```python
from build123d import *
from build123d.topology import SkipClean

# Parameters (mm, degrees)
EXTRUDE1_DEPTH  = 21.397127
SKETCH4_W       = 60
SKETCH4_H       = 29.397126503
SKETCH3_W       = 80
SKETCH3_H       = 20
EXTRUDE2_DEPTH  = 10
EXTRUDE3_DEPTH  = 9
SKETCH7_W       = 60.014196904
SKETCH7_H       = 26.778889024
EXTRUDE4_DEPTH  = 11
SKETCH8_W       = 71.467077652
SKETCH8_H       = 25.017155062
EXTRUDE5_DEPTH  = 23
SKETCH9_W       = 59.977554146
SKETCH9_H       = 30.874003366
EXTRUDE6_DEPTH  = 7
SKETCH10_R      = 2.5
EXTRUDE7_DEPTH  = 65
SKETCH12_R      = 5
EXTRUDE8_DEPTH  = 65
SKETCH13_R      = 2.15
EXTRUDE9_DEPTH  = 65
SKETCH14_R      = 4
EXTRUDE10_DEPTH = 65


with BuildPart() as part:
    # Sketch1 → Extrude1 (new body)
    with BuildSketch(Plane.XY):
        with BuildLine():
            Line((-96.138674094, 82.333988555), (-46.138674094, 82.333988555))
            Line((-46.138674094, 82.333988555), (-46.138674094, 131.333988555))
            ThreePointArc((-46.138674094, 131.333988555), (-47.017353751, 133.455308898), (-49.138674094, 134.333988555))
            Line((-49.138674094, 134.333988555), (-93.138674094, 134.333988555))
            ThreePointArc((-93.138674094, 134.333988555), (-95.259994438, 133.455308898), (-96.138674094, 131.333988555))
            Line((-96.138674094, 131.333988555), (-96.138674094, 82.333988555))
        make_face()
        with BuildLine():
            ThreePointArc((-86.138674094, 92.833988555), (-83.638674094, 95.333988555), (-86.138674094, 97.833988555))
            ThreePointArc((-86.138674094, 97.833988555), (-88.638674094, 95.333988555), (-86.138674094, 92.833988555))
        make_face(mode=Mode.SUBTRACT)
        with BuildLine():
            ThreePointArc((-56.138674094, 92.833988555), (-53.638674094, 95.333988555), (-56.138674094, 97.833988555))
            ThreePointArc((-56.138674094, 97.833988555), (-58.638674094, 95.333988555), (-56.138674094, 92.833988555))
        make_face(mode=Mode.SUBTRACT)
        with BuildLine():
            ThreePointArc((-86.138674094, 127.833988555), (-88.638674094, 125.333988555), (-86.138674094, 122.833988555))
            ThreePointArc((-86.138674094, 122.833988555), (-83.638674094, 125.333988555), (-86.138674094, 127.833988555))
        make_face(mode=Mode.SUBTRACT)
        with BuildLine():
            ThreePointArc((-56.138674094, 122.833988555), (-53.638674094, 125.333988555), (-56.138674094, 127.833988555))
            ThreePointArc((-56.138674094, 127.833988555), (-58.638674094, 125.333988555), (-56.138674094, 122.833988555))
        make_face(mode=Mode.SUBTRACT)
        with BuildLine():
            ThreePointArc((-71.138674094, 125.333988555), (-86.138674094, 110.333988555), (-71.138674094, 95.333988555))
            ThreePointArc((-71.138674094, 95.333988555), (-56.138674094, 110.333988555), (-71.138674094, 125.333988555))
        make_face(mode=Mode.SUBTRACT)
    extrude(amount=EXTRUDE1_DEPTH)

    # Sketch4 → Loft1 section 0
    with BuildSketch(Plane(origin=(0, 117.333988555, 0), x_dir=(1, 0, 0), z_dir=(0, 1, 0))):
        with Locations((-71.138674094, -14.698563252)):
            Rectangle(SKETCH4_W, SKETCH4_H)
    # Sketch3 → Loft1 section 1
    with BuildSketch(Plane(origin=(0, 102.333988555, 0), x_dir=(1, 0, 0), z_dir=(0, 1, 0))):
        with Locations((-71.138674094, -31.397126503)):
            Rectangle(SKETCH3_W, SKETCH3_H)
    loft()

    # Sketch5 → Extrude2 (add)
    with BuildSketch(Plane(origin=(25.673528037, 17.115685358, 0), x_dir=(0, 0, -1), z_dir=(0.8320502943378439, 0.5547001962252289, 0))):
        Polygon((-29.397126503, 120.447410305), (-15.115551494, 141.902806552), (0, 141.902806552), (0, 120.447410305), align=None)
    extrude2 = extrude(amount=-EXTRUDE2_DEPTH)

    # Mirror1: Extrude2 across plane
    add(extrude2.mirror(Plane(origin=(-71.138674094, 0, 0), x_dir=(0, 0, 1), z_dir=(1, 0, 0))))

    # Sketch6 → Extrude3 (add)
    with BuildSketch(Plane(origin=(0, 60.128935291, 75.161169114), x_dir=(1, 0, 0), z_dir=(0, 0.6246950475544204, 0.7808688094430335))):
        Polygon((-101.138674094, 73.258212611), (-85.265778398, 103.749049557), (-57.011569791, 103.749049557), (-41.138674094, 73.258212611), align=None)
    extrude(amount=-EXTRUDE3_DEPTH)

    # Sketch7 → Extrude4 (cut)
    with BuildSketch(Plane(origin=(0, 60.128935291, 75.161169114), x_dir=(1, 0, 0), z_dir=(0, 0.6246950475544204, 0.7808688094430335))):
        with Locations((-68.308122793, 89.258337759)):
            Rectangle(SKETCH7_W, SKETCH7_H)
    extrude(amount=EXTRUDE4_DEPTH, mode=Mode.SUBTRACT)

    # Sketch8 → Extrude5 (cut)
    with BuildSketch(Plane(origin=(-124.173230629, 82.782153753, 0), x_dir=(0, 0, 1), z_dir=(-0.8320502943378424, 0.554700196225231, 1.5396023240333535e-15))):
        with Locations((13.757489511, 55.477649782)):
            Rectangle(SKETCH8_W, SKETCH8_H)
    extrude5 = extrude(amount=EXTRUDE5_DEPTH, mode=Mode.SUBTRACT)

    # Mirror2: Extrude5 across plane
    add(extrude5.mirror(Plane(origin=(-71.138674094, 0, 0), x_dir=(0, 0, 1), z_dir=(1, 0, 0))), mode=Mode.SUBTRACT)

    # Sketch9 → Extrude6 (cut)
    with BuildSketch(Plane(origin=(0, 134.333988555, 0), x_dir=(1, 0, 0), z_dir=(0, 1, 0))):
        with Locations((-70.004468298, -10.685148069)):
            Rectangle(SKETCH9_W, SKETCH9_H)
    extrude(amount=EXTRUDE6_DEPTH, mode=Mode.SUBTRACT)

    # Sketch10 → Extrude7 (cut)
    with SkipClean():  # the faces are left unmerged after this step: merging them gives an invalid solid
        with BuildSketch(Plane(origin=(0, 0, 0), x_dir=(-1, 0, 0), z_dir=(0, 0, -1))):
            with BuildLine():
                ThreePointArc((84.405173256, 117.333988555), (71.138674094, 125.333988555), (57.872174933, 117.333988555))
                ThreePointArc((57.872174933, 117.333988555), (56.149794828, 109.756495394), (58.450096554, 102.333988555))
                ThreePointArc((58.450096554, 102.333988555), (78.644238587, 97.346821748), (84.405173256, 117.333988555))
            make_face()
            with Locations(Location((56.138674094, 125.333988555, 0), (0, 0, 90))):
                Circle(SKETCH10_R)
            with Locations(Location((86.138674094, 125.333988555, 0), (0, 0, 90))):
                Circle(SKETCH10_R)
        extrude(amount=-EXTRUDE7_DEPTH, mode=Mode.SUBTRACT)

    # Sketch12 → Extrude8 (cut)
    with SkipClean():  # the faces are left unmerged after this step: merging them gives an invalid solid
        with BuildSketch(Plane(origin=(0, 0, 8), x_dir=(-1, 0, 0), z_dir=(0, 0, -1))):
            with Locations((86.138674094, 125.333988555)):
                Circle(SKETCH12_R)
            with Locations((56.138674094, 125.333988555)):
                Circle(SKETCH12_R)
        extrude(amount=-EXTRUDE8_DEPTH, mode=Mode.SUBTRACT)

    # Sketch13 → Extrude9 (cut)
    with BuildSketch(Plane.XZ.offset(-102.333988555)):
        with Locations(Location((-104.138674094, 31.397126503, 0), (0, 0, 270))):
            Circle(SKETCH13_R)
        with Locations(Location((-90.827251635, 31.397126503, 0), (0, 0, 270))):
            Circle(SKETCH13_R)
        with Locations(Location((-51.450096554, 31.397126503, 0), (0, 0, 270))):
            Circle(SKETCH13_R)
        with Locations(Location((-38.138674094, 31.397126503, 0), (0, 0, 270))):
            Circle(SKETCH13_R)
    extrude(amount=-EXTRUDE9_DEPTH, mode=Mode.SUBTRACT)

    # Sketch14 → Extrude10 (cut)
    with BuildSketch(Plane(origin=(0, 108.333988555, 0), x_dir=(-1, 0, 0), z_dir=(0, -1, 0))):
        with Locations((104.138674094, -31.397126503)):
            Circle(SKETCH14_R)
        with Locations(Location((90.827251635, -31.397126503, 0), (0, 0, 90))):
            Circle(SKETCH14_R)
        with Locations(Location((51.450096554, -31.397126503, 0), (0, 0, 90))):
            Circle(SKETCH14_R)
        with Locations((38.138674094, -31.397126503)):
            Circle(SKETCH14_R)
    extrude(amount=-EXTRUDE10_DEPTH, mode=Mode.SUBTRACT)


solid = part.part
```
Build history of the part. All positions in model axes, mm. A direction names the side the tool comes from. Round coordinates to 2 decimals unless told otherwise and drop trailing zeros. Loops run counter-clockwise (first coordinate to the right, second up) from the corner with the lowest first, then second, coordinate; pieces in that order, holes last.
Item 1: Saw through at A-A (x = -72.5). List the corners of the cut face in (y, z).
Item 2: Saw through at C-C (z = 26). List the corners of the cut face in (x, y).
Item 3: Drill centre lines: line 1 along Y through (x, z) = (-59, 17.5); line 2 along X through (y, z) = (92.5, 2); line 3 along X through (y, z) = (110.5, 29.5). Where is each one in solid material? Low to high.
Item 4: Saw through at B-B (y = 99). List the corners of the cut face in (x, z).
Item 5: Two-plate mould, pull along Z, no slides. Class faces 4 (the face through (-83.92, 96.49, 10.55)), 5 (the face through (-41.642, 110.878, 29.467)), 6 (the face through (-87, 128, 8)): released by +Z, released by -Z, zero draft, split by the parting line, or undercut.
Item 6: Saw through at D-D (x = -63.5). List the corners of the cut face in (y, z), then the cut area to 3 significant figures.
Item 7: Pin check, flat tips, straight feed: P1, Ø2, axis at x = -48.5, y = 93.5, coming from the +Z side; P2, Ø4, axis at y = 113.5, z = 14, coming from the +X side; P3, Ø13, axis at x = -90.83, z = 31.4, coming from the -Y side. Stop position of each tip, or through.
Item 8: Which spindle directions (+Z, -Z, +X, -X, +Y, -Y) get a long thin tool onto all of the face, cutting with end or side? Do faces 1 (the face through (-85.055, 120.453, 15.291)), 2 (the face through (-45, 102.334, 31)), 3 (the face through (-89.63, 112.73, 27.58)). Say none if no direction does.
Worked answers:
1. outline: (82.33, 0) - (95.4, 0) - (95.4, 21.4) - (82.33, 21.4) - close; (125.27, 0) - (134.33, 0) - (134.33, 15.8) - (125.27, 23.05) - close
2. outline: (-111.14, 102.33) - (-83.83, 102.33) arc R15 cw to (-81.06, 121.58) - (-82.84, 121.58) arc R5 cw to (-89.44, 121.58) - (-98.31, 121.58) - close; (-61.21, 121.58) arc R15 cw to (-58.45, 102.33) - (-31.14, 102.33) - (-43.97, 121.58) - (-52.84, 121.58) arc R5 cw to (-59.44, 121.58) - close
3. line 1: y = 82.33 to 101.52, 119.15 to 121.23, 129.43 to 132.21
3. line 2: x = -96.14 to -46.14
3. line 3: x = -100.62 to -94.35, -87.31 to -86.14, -56.14 to -54.97, -47.93 to -41.66
4. outline: (-96.14, 0) - (-80.96, 0) - (-80.96, 21.4) - (-96.14, 21.4) - close; (-61.31, 0) - (-46.14, 0) - (-46.14, 21.4) - (-61.31, 21.4) - close
5. face 4: zero draft
5. face 5: undercut
5. face 6: released by +Z
6. outline: (82.33, 0) - (97.42, 0) - (97.42, 21.4) - (82.33, 21.4) - close; (123.24, 0) - (134.33, 0) - (134.33, 15.8) - (123.24, 24.67) - close
6. area: 547 mm2
7. P1: stops at z = 21.4
7. P2: stops at x = -37.25
7. P3: stops at y = 102.33
8. face 1: +Z
8. face 2: +Z, +X, -X, -Y
8. face 3: +Y
